Check sheet for the modelled part. Datum: model origin and axes. Units: mm. Give positions to 0.01 mm unless a question says otherwise; leave off trailing zeros. Order: outer loops, then holes, each group sorted by start corner. A loop starts at its lowest first (then second) coordinate and runs counter-clockwise, first axis right, second up. Notation, with made-up numbers: M -1,35.5 L 54,35.5 A19 cw 54,59.5 Z; hole C 87.25,31 d8. An arc over 180 degrees is marked long. One line per question, with ' | ' between items. Start each with the question number.
```python
from build123d import *

# Parameters (mm, degrees)
SKETCH1_R           = 4.5
SKETCH1_R_2         = 2.5
BOSS_EXTRUDE1_DEPTH = 11
SKETCH2_R           = 2
CHAMFER1_SIZE       = 0.635
CHAMFER2_SIZE       = 0.254


with BuildPart() as part:
    # Sketch1 → Boss-Extrude1 (new body)
    with BuildSketch(Plane.XY):
        Circle(SKETCH1_R)
        Circle(SKETCH1_R_2, mode=Mode.SUBTRACT)
    extrude(amount=BOSS_EXTRUDE1_DEPTH)

    # Sketch2 → Cut-Revolve1 (revolve, cut)
    with BuildSketch(Plane(origin=(0, 0, 0), x_dir=(-1, 0, 0), z_dir=(0, -1, 0)), mode=Mode.PRIVATE) as cut_revolve1_sk:
        with Locations((5.822875656, -8.484)):
            Circle(SKETCH2_R)
    revolve(cut_revolve1_sk.sketch.rotate(Axis((0, 0, 11), (0, 0, -1)), 180), axis=Axis((0, 0, 11), (0, 0, -1)), mode=Mode.SUBTRACT)

    # Chamfer1
    chamfer1_edges = [part.edges().sort_by_distance(p)[0] for p in [
        (-4.5, 0, 11),
    ]]
    chamfer(chamfer1_edges, length=CHAMFER1_SIZE)

    # Chamfer2
    chamfer2_edges = [part.edges().sort_by_distance(p)[0] for p in [
        (-4.5, 0, 0),
        (-2.5, 0, 0),
        (-2.5, 0, 11),
    ]]
    chamfer(chamfer2_edges, length=CHAMFER2_SIZE)


solid = part.part
```
Item 1: Scan lines: probe 1 along Y at (x, z) = (0, 5.5); probe 2 along Y at (x, z) = (0, 7.25); probe 3 along X at (y, z) = (-1.25, 3.5). Record each from-to range of solid material in increasing order. Write a range as [from, to].
Item 2: Go/stop test with flat-tipped pins: P1, Ø3, axis at y = 0.5, z = 6.5, coming from the +X side; P2, Ø4, axis at y = -2.5, z = 3, coming from the -X side. Record where each tip stops, or that it passes through.
Item 3: Section check C-C, the plane z = 5.25. Record the cut outline in (x, y).
Item 4: Draft check along X on faces 1 (the face through (-0.59, 4.46, 10.17)), 2 (the face through (-1, 3, 11)), 3 (the face through (-0.54, -2.44, 5.43)). Enter one of: released by +X, released by -X, zero draft, split by the parting line, or undercut.
Item 5: Section check A-A, the plane y = 0. Record the cut outline in (x, z) (3 decimals), then the cut area to 3 significant figures.
Reported:
1) probe 1: y = [-4.5, -2.5], [2.5, 4.5] | probe 2: y = [-4.25, -2.5], [2.5, 4.25] | probe 3: x = [-4.32, -2.17], [2.17, 4.32]
2) P1: stops at x = 4.5 | P2: stops at x = -4.47
3) outline: C 0,0 d9; hole C 0,0 d5
4) face 1: split by the parting line | face 2: zero draft | face 3: undercut
5) outline: M -4.5,0.254 L -4.246,0 L -2.754,0 L -2.5,0.254 L -2.5,10.746 L -2.754,11 L -3.865,11 L -4.5,10.365 L -4.5,9.984 A2 cw -4.5,6.984 Z; M 2.5,0.254 L 2.754,0 L 4.246,0 L 4.5,0.254 L 4.5,6.984 A2 cw 4.5,9.984 L 4.5,10.365 L 3.865,11 L 2.754,11 L 2.5,10.746 Z | area: 40.6 mm^2
